CAD build for the part. Positions are in the model's coordinates, mm. Face numbers are marked on the shaded views. A direction names the side the tool comes from. Round coordinates to 2 decimals unless told otherwise and drop trailing zeros. Write each loop counter-clockwise with the first axis right and the second up, starting at its lowest first coordinate (ties: lowest second). Pieces come first, ordered by that corner, then holes. Notation, with made-up numbers: (25.5, 73) - (69.5, 73) arc R19 ccw to (69.5, 82) - close; hole circle Ø2 at (29, 6.5). An arc over 180 degrees is marked (long way). Use one line per item in the form item = value. Start each with the question number.
Item 1: Drill centre lines: L1, parallel to Y at x = 0, z = 9.5; L2, parallel to X at y = 5, z = 14; L3, parallel to X at y = -1.5, z = 13. Where is each one in solid material? Low to high.
Item 2: Pull direction X, two halves, no side cores. Call the marked faces 4, 5, 6 and 7: +X half, -X half, draft (parallel to the pull), parting line (faces both ways), or undercut.
Item 3: Band-saw the part on C-C, the plane x = 0. List the corners of the cut face in (y, z).
Item 4: Band-saw the part on B-B, the plane z = 7.5. List the corners of the cut face in (x, y).
Item 5: Band-saw the part on D-D, the plane y = -24.5. List the corners of the cut face in (x, z), and give its area (3 significant figures).
Item 6: Band-saw the part on A-A, the plane y = 0. List the corners of the cut face in (x, z).
Item 7: Tool access for the marked faces 1, 2 and 3: list every direction of +Z, -Z, +X, -X, +Y, -Y with a clear straight run to the whole face (end or side of a thin tool).
Item 8: Pin check, flat tips, straight feed: pin 1 (4.5 mm diameter, centred on x = 1, y = -24.5, fed in from +Z); pin 2 (0.9 mm diameter, centred on y = 17.5, z = 14, fed in from +X). Stop position of each tip, or through.
from build123d import *

# Parameters (mm, degrees)
F0_W     = 100
F0_H     = 60
F0_R     = 12.5
F1_DEPTH = 15
F2_W     = 10
F2_H     = 60
F3_DEPTH = 3
F5_DEPTH = 60.001
F6_R     = 5
F7_DEPTH = 15


with BuildPart() as f1:
    # F0 (on Top) → F1 (new body)
    with BuildSketch(Plane.XY):
        Rectangle(F0_W, F0_H)
        Circle(F0_R, mode=Mode.SUBTRACT)
    extrude(amount=F1_DEPTH)

    # F2 (on face) → F3 (cut)
    with BuildSketch(Plane.XY.offset(15)):
        with BuildLine():
            Line((7.5, 30), (-7.5, 30))
            Line((-7.5, 30), (-7.5, 10))
            ThreePointArc((-7.5, 10), (0, 12.5), (7.5, 10))
            Line((7.5, 10), (7.5, 30))
        make_face()
        with BuildLine():
            Line((-7.5, -10), (-7.5, -30))
            Line((-7.5, -30), (7.5, -30))
            Line((7.5, -30), (7.5, -10))
            ThreePointArc((7.5, -10), (0, -12.5), (-7.5, -10))
        make_face()
        with Locations((-40, 0)):
            Rectangle(F2_W, F2_H)
    extrude(amount=-F3_DEPTH, mode=Mode.SUBTRACT)

    # F4 (on face) → F5 (cut, through all)
    with BuildSketch(Plane.XZ.offset(30)):
        Polygon((30, 15), (20, 15), (17.5, 10.669873), (32.5, 10.669873), align=None)
    extrude(amount=-F5_DEPTH, mode=Mode.SUBTRACT)

    # F6 (on face) → F7 (join)
    with BuildSketch(Plane.YZ.offset(50)):
        with Locations((0, 7.5)):
            Circle(F6_R)
    extrude(amount=F7_DEPTH)


solid = f1.part
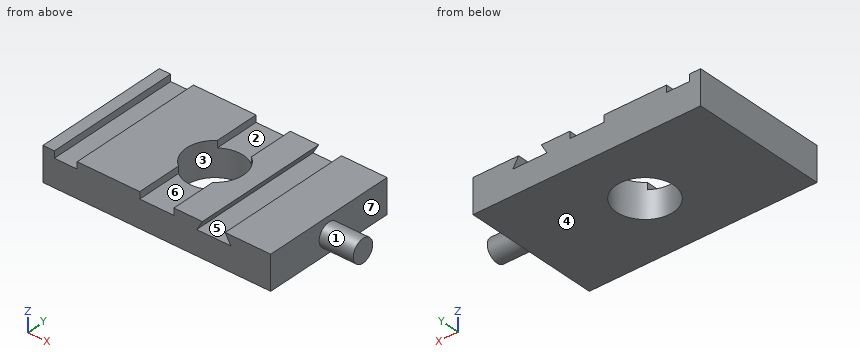
Determined:
q1.L1 = -30 to -12.5, 12.5 to 30
q1.L2 = -50 to -45, -35 to -11.46, 11.46 to 19.42, 30.58 to 50
q1.L3 = -50 to -45, -35 to -12.41, 12.41 to 18.85, 31.15 to 50
q2.face_4 = draft
q2.face_5 = undercut
q2.face_6 = undercut
q2.face_7 = +X half
q3.outline = (-30, 0) - (-12.5, 0) - (-12.5, 12) - (-30, 12) - close; (12.5, 0) - (30, 0) - (30, 12) - (12.5, 12) - close
q4.outline = (-50, -30) - (50, -30) - (50, -5) - (65, -5) - (65, 5) - (50, 5) - (50, 30) - (-50, 30) - close; hole circle Ø25 at (0, 0)
q5.outline = (-50, 0) - (50, 0) - (50, 15) - (30, 15) - (32.5, 10.67) - (17.5, 10.67) - (20, 15) - (7.5, 15) - (7.5, 12) - (-7.5, 12) - (-7.5, 15) - (-35, 15) - (-35, 12) - (-45, 12) - (-45, 15) - (-50, 15) - close
q5.area = 1,370 mm²
q6.outline = (-50, 0) - (-12.5, 0) - (-12.5, 15) - (-35, 15) - (-35, 12) - (-45, 12) - (-45, 15) - (-50, 15) - close; (12.5, 0) - (50, 0) - (50, 2.5) - (65, 2.5) - (65, 12.5) - (50, 12.5) - (50, 15) - (30, 15) - (32.5, 10.67) - (17.5, 10.67) - (20, 15) - (12.5, 15) - close
q7.face_1 = +X
q7.face_2 = +Z, +Y, -Y
q7.face_3 = +Z, -Z
q8.pin_1 = 12
q8.pin_2 = 50
